Autodesk Inventor part; units mm, degrees
ref_plane "YZ Plane" through (0, 0, 0) normal (1, 0, 0) x (0, 1, 0)
ref_plane "XZ Plane" through (0, 0, 0) normal (0, 1, 0) x (-1, 0, 0)
ref_plane "XY Plane" through (0, 0, 0) normal (0, 0, 1) x (1, 0, 0)
sketch "スケッチ1" plane through (0, 0, 0) normal (0, 0, 1) x (1, 0, 0)
  line L0 (0, 0) -> (-26.8716, 23) construction
  line L1 (32.7705, -12.2921) -> (0, 0) construction
  circle A0 centre (0, 0) radius 8
  circle A1 centre (0, 0) radius 6.025
  circle A2 centre (0, 0) radius 10
  line L2 (30.3398, -14.0505) -> (4.0407, -9.1473)
  line L3 (9.0597, 4.2333) -> (32.0958, -9.369)
  line L4 (-23.9861, 23.821) -> (-0.5538, 9.9847)
  line L5 (-9.9505, -0.9938) -> (-27.2374, 20.0224)
  circle A3 centre (-10.7763, 6.3341) radius 3.05
  circle A4 centre (-10.7763, 6.3341) radius 1.25
  circle A5 centre (10.7763, -6.3341) radius 3.05
  circle A6 centre (10.7763, -6.3341) radius 1.25
  arc A7 (-10.6465, 10.3494) -> (-13.8789, 3.7821) centre (-10.7763, 6.3341) ccw
  arc A8 (10.0432, -10.2664) -> (14.2097, -4.2819) centre (10.7763, -6.3341) ccw
  line L6 (-10.6465, 10.3494) -> (0.3231, 9.9948)
  line L7 (8.5835, 5.1307) -> (14.2097, -4.2819)
  line L8 (10.0432, -10.2664) -> (-0.2617, -9.9966)
  line L9 (-8.5971, -5.1078) -> (-13.8789, 3.7821)
  point P0 (-0.6227, 10.0254)
  point P1 (9.1526, 4.1785)
  dimension "d0" = 12.05
  dimension "d5" = 2.5
extrude "押し出し1" add sketch "スケッチ1" along normal blind 3 contours A0 | A2 A5 A3 | A2 L3 L7 A8 L2 A5 | A5 A2 | A2 A5 | L2 L8 A2 | A2 A3 L5 A7 L6 L4 | A3 A2 | A2 A3 | L9 L5 A2
extrude "押し出し2" cut sketch "スケッチ1" along normal blind 1 contours A5 A2 | A2 A5 | A3 A2 | A2 A3 | A4 | A6
properties part number "モータマウント2" material "アルミニウム 2014-T4"
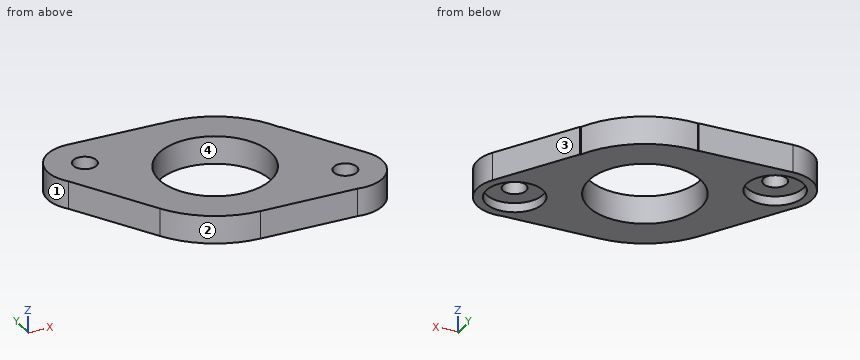
Verification items for the finished model (mm, model axes). Face numbers are marked on the shaded views. Give positions to 0.01 mm unless a question says otherwise; leave off trailing zeros. Order: outer loops, then holes, each group sorted by start corner. A loop starts at its lowest first (then second) coordinate and runs counter-clockwise, first axis right, second up. Notation, with made-up numbers: M 30.5,77.25 L 59.5,77.25 A19 cw 59.5,93.25 Z; hole C 21.5,64.5 d7. An arc over 180 degrees is marked long. Return JSON: item names as keys, results as strings. Group by question number.
1) Section check D-D on x = -11. Record the cut outline in (y, z), and give its area (3 significant figures).
2) Section check C-C on z = 1.75. Give the number of separate pieces and of enclosed holes in the cut face, and give its area (3 significant figures).
3) Section check A-A on y = 2.5. Record the cut outline in (x, z).
4) Go/stop test with flat-tipped pins: pin 1 Ø4 at (x, y) = (-10.78, 6.33) entering from +Z; pin 2 Ø3.5 at (x, y) = (10.78, -6.33) entering from -Z; pin 3 Ø9.5 at (x, y) = (0, 0) entering from +Z; pin 4 Ø1 at (x, z) = (-8, 1.5) entering from -Y. Record where each tip stops, or that it passes through.
5) Section check B-B on x = 10.5. Record the cut outline in (y, z).
6) Scan lines: line 1 (Y direction, x = 0, z = 0.75) (3 decimals); line 2 (X direction, y = -0.75, z = 1.2); line 3 (X direction, y = 3.25, z = 2.65). Record each from-to range of solid material in increasing order.
7) Mould release check, pull along Y, two halves, no side actions. Record for the marked faces 1, 2, 3 and 4: pulls with the +Y half, pulls with the -Y half, needs draft (parallel to the pull), parting line crosses it, or undercut.
Answer block:
{
 "1": {"outline": "M -1.06,0 L 3.29,0 L 3.29,1 L 5.1,1 L 5.1,3 L -1.06,3 Z; M 7.56,1 L 9.38,1 L 9.38,0 L 10.35,0 L 10.35,3 L 7.56,3 Z", "area": "23.2 mm^2"},
 "2": {"separate pieces": "1", "enclosed holes": "3", "area": "317 mm^2"},
 "3": {"outline": "M -13.12,0 L -5.48,0 L -5.48,3 L -13.12,3 Z; M 5.48,0 L 10.16,0 L 10.16,3 L 5.48,3 Z"},
 "4": {"pin 1": "stops at z = 3", "pin 2": "stops at z = 1", "pin 3": "passes through", "pin 4": "stops at y = -6.61"},
 "5": {"outline": "M -10.32,0 L -9.37,0 L -9.37,1 L -7.55,1 L -7.55,3 L -10.32,3 Z; M -5.12,1 L -3.3,1 L -3.3,0 L 1.92,0 L 1.92,3 L -5.12,3 Z"},
 "6": {"line 1": "y = -10.003 to -6.025, 6.025 to 10", "line 2": "x = -11.19 to -5.98, 5.98 to 12.1", "line 3": "x = -13.56 to -5.07, 5.07 to 9.71"},
 "7": {"face 1": "parting line crosses it", "face 2": "pulls with the -Y half", "face 3": "pulls with the +Y half", "face 4": "undercut"}
}
